```python
from build123d import *

# Parameters (mm, degrees)
BOSS_EXTRU_1_DEPTH      = 5
ESQUISSE2_R             = 7
BOSS_EXTRU_2_DEPTH      = 15
ESQUISSE3_R             = 5
ENL_V_MAT_EXTRU_1_DEPTH = 30
ESQUISSE4_R             = 2.25
ENL_V_MAT_EXTRU_2_DEPTH = 30


with BuildPart() as part:
    # Esquisse1 → Boss.-Extru.1 (new body)
    with BuildSketch(Plane(origin=(0, 0, 0), x_dir=(1, 0, 0), z_dir=(0, 1, 0))):
        with BuildLine():
            Line((-9, 12), (-9, -12))
            ThreePointArc((-9, -12), (0, -15), (9, -12))
            Line((9, -12), (9, 12))
            ThreePointArc((9, 12), (0, 15), (-9, 12))
        make_face()
    extrude(amount=BOSS_EXTRU_1_DEPTH)

    # Esquisse2 → Boss.-Extru.2 (add)
    with BuildSketch(Plane(origin=(0, 5, 0), x_dir=(1, 0, 0), z_dir=(0, 1, 0))):
        with Locations(Location((0, 0, 0), (0, 0, 270))):
            Circle(ESQUISSE2_R)
    extrude(amount=BOSS_EXTRU_2_DEPTH)

    # Esquisse3 → Enlèv. mat.-Extru.1 (cut)
    with BuildSketch(Plane(origin=(0, 20, 0), x_dir=(1, 0, 0), z_dir=(0, 1, 0))):
        with Locations(Location((0, 0, 0), (0, 0, 270))):
            Circle(ESQUISSE3_R)
    extrude(amount=-ENL_V_MAT_EXTRU_1_DEPTH, mode=Mode.SUBTRACT)

    # Esquisse4 → Enlèv. mat.-Extru.2 (cut)
    with BuildSketch(Plane(origin=(0, 5, 0), x_dir=(1, 0, 0), z_dir=(0, 1, 0))):
        with Locations(Location((0, 11, 0), (0, 0, 270))):
            Circle(ESQUISSE4_R)
        with Locations(Location((0, -11, 0), (0, 0, 270))):
            Circle(ESQUISSE4_R)
    extrude(amount=-ENL_V_MAT_EXTRU_2_DEPTH, mode=Mode.SUBTRACT)


solid = part.part
```
CAD build for the part. Positions are in the model's coordinates, mm. A direction names the side the tool comes from. Round coordinates to 2 decimals unless told otherwise and drop trailing zeros. Loops run counter-clockwise (first coordinate to the right, second up) from the corner with the lowest first, then second, coordinate; pieces in that order, holes last. Notation, with made-up numbers: (50.5, 72) - (74.5, 72) arc R12 cw to (74.5, 86) - close; hole circle Ø5 at (7.25, 54). An arc over 180 degrees is marked (long way). Return JSON: item names as keys, results as strings. Group by question number.
Q1. Tool access for faces 5 (the face through (0.099, 2.535, 8.752)), 6 (the face through (-2, 5, -7)): list every direction of +Z, -Z, +X, -X, +Y, -Y with a clear straight run to the whole face (end or side of a thin tool).
Q2. Band-saw the part on D-D on x = -4. Give the cut face in (y, z), plus the area to 3 significant figures.
Q3. Band-saw the part on C-C on y = 2. Give the cut face in (x, z).
Q4. Flat gauge pins, fed straight in: pin 1 Ø6 at (x, y) = (-7, 4) entering from -Z; pin 2 Ø1 at (y, z) = (7.5, 5.5) entering from -X; pin 3 Ø2 at (x, y) = (3, 5) entering from -Z. Where does each tip first touch, or does it go through?
Q5. Band-saw the part on B-B on z = -11. Give the cut face in (x, y), plus the area to 3 significant figures.
Q6. Band-saw the part on A-A on x = 0. Give the cut face in (y, z), plus the area to 3 significant figures.
Q7. Two-plate mould, pull along X, no slides. Class faces 1 (the face through (-4.88, 10.14, -1.08)), 2 (the face through (0.099, 2.535, -13.248)), 3 (the face through (5, 20, -2)), 4 (the face through (9, 2, 0)): +X half, -X half, draft (parallel to the pull), parting line (faces both ways), or undercut.
Q8. Drill centre lines: line 1 along X through (y, z) = (1.5, -11); line 2 along Z through (x, y) = (-1.75, 3); line 3 along Y through (x, z) = (3.25, -9.75). Where is each one in solid material? Low to high. Write a range as [from, to].
Solutions:
{
 "1": {"face 5": "+Y, -Y", "face 6": "+Y"},
 "2": {"outline": "(0, -14.46) - (5, -14.46) - (5, -5.74) - (20, -5.74) - (20, -3) - (0, -3) - close; (0, 3) - (20, 3) - (20, 5.74) - (5, 5.74) - (5, 14.46) - (0, 14.46) - close", "area": "197 mm^2"},
 "3": {"outline": "(-9, -12) arc R15 ccw to (9, -12) - (9, 12) arc R15 ccw to (-9, 12) - close; hole circle Ø10 at (0, 0); hole circle Ø4.5 at (0, -11); hole circle Ø4.5 at (0, 11)"},
 "4": {"pin 1": "stops at z = -14.46", "pin 2": "stops at x = -4.9", "pin 3": "stops at z = -14.87"},
 "5": {"outline": "(-9, 0) - (-2.25, 0) - (-2.25, 5) - (-9, 5) - close; (2.25, 0) - (9, 0) - (9, 5) - (2.25, 5) - close", "area": "67.5 mm^2"},
 "6": {"outline": "(0, -15) - (5, -15) - (5, -13.25) - (0, -13.25) - close; (0, -8.75) - (5, -8.75) - (5, -7) - (20, -7) - (20, -5) - (0, -5) - close; (0, 5) - (20, 5) - (20, 7) - (5, 7) - (5, 8.75) - (0, 8.75) - close; (0, 13.25) - (5, 13.25) - (5, 15) - (0, 15) - close", "area": "115 mm^2"},
 "7": {"face 1": "undercut", "face 2": "undercut", "face 3": "draft", "face 4": "+X half"},
 "8": {"line 1": "x = [-9, -2.25], [2.25, 9]", "line 2": "z = [-14.9, -12.41], [-9.59, -4.68], [4.68, 9.59], [12.41, 14.9]", "line 3": "y = [0, 5]"}
}
